Here's how the part is built. I have some questions about the finished solid (model axes, mm). Give positions to 0.01 mm unless a question says otherwise; leave off trailing zeros. Loops run counter-clockwise (first coordinate to the right, second up) from the corner with the lowest first, then second, coordinate; pieces in that order, holes last.
Q1. Suppose I cut it at B-B (z = -177.8). List the corners of the cut face in (x, y) for me, and give its area (3 significant figures).
Q2. Suppose I cut it at A-A (x = 2.75). Count the separate pieces of the cut face and the enclosed holes in it, and give its area (3 significant figures).
Q3. I'm going to push a flat-ended pin straight in: P1, Ø2, axis at x = 5, y = 36.5, coming from the -Z side. Where does the tip first touch, or does it pass through?
Q4. I need wall thicknesses on probe 1 along Y at (x, z) = (4.25, -355.6); probe 2 along Y at (x, z) = (3.75, -25.4); probe 3 along Z at (x, y) = (2.5, 15.5). Which ranges of each line are inside material? Lowest first, please.
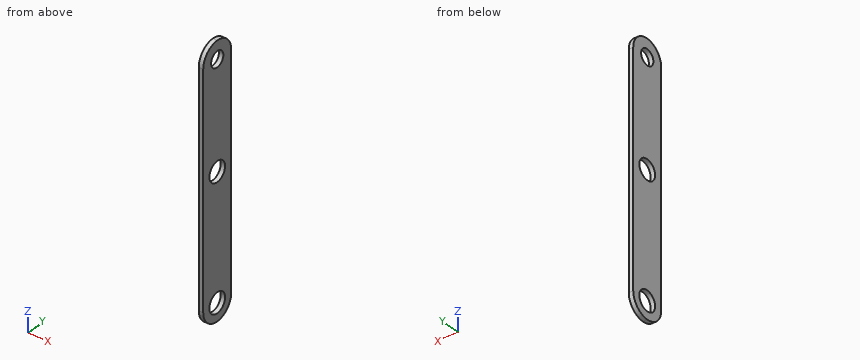
```python
from build123d import *

# Parameters (mm, degrees)
SKETCH1_W           = 381
SKETCH1_H           = 50.8
SKETCH1_R           = 11.1125
SKETCH1_R_2         = 14.2875
BOSS_EXTRUDE1_DEPTH = 6.35
FILLET3_R           = 25.4


with BuildPart() as part:
    # Sketch1 → Boss-Extrude1 (new body)
    with BuildSketch(Plane(origin=(0, 0, 0), x_dir=(0, 0, -1), z_dir=(1, 0, 0))):
        with Locations((190.5, 25.4)):
            Rectangle(SKETCH1_W, SKETCH1_H)
        with Locations((25.4, 25.4)):
            Circle(SKETCH1_R, mode=Mode.SUBTRACT)
        with Locations(Location((355.6, 25.4, 0), (0, 0, 180))):
            Circle(SKETCH1_R_2, mode=Mode.SUBTRACT)
        with Locations((177.8, 25.4)):
            Circle(SKETCH1_R_2, mode=Mode.SUBTRACT)
    extrude(amount=BOSS_EXTRUDE1_DEPTH)

    # Fillet3
    fillet3_edges = [part.edges().sort_by_distance(p)[0] for p in [
        (3.175, 0, 0),
        (3.175, 50.8, 0),
        (3.175, 0, -381),
        (3.175, 50.8, -381),
    ]]
    fillet(fillet3_edges, radius=FILLET3_R - 0.0001)  # a hair under: the kernel refuses the full size


solid = part.part
```
Solutions:
1. outline: (0, 0) - (6.35, 0) - (6.35, 11.11) - (0, 11.11) - close; (0, 39.69) - (6.35, 39.69) - (6.35, 50.8) - (0, 50.8) - close
1. area: 141 mm2
2. separate pieces: 1
2. enclosed holes: 3
2. area: 17,100 mm2
3. P1: stops at z = -378.91
4. probe 1: y = 0 to 11.11, 39.69 to 50.8
4. probe 2: y = 0 to 14.29, 36.51 to 50.8
4. probe 3: z = -378.99 to -365.9, -345.3 to -188.1, -167.5 to -30.45, -20.35 to -2.01
